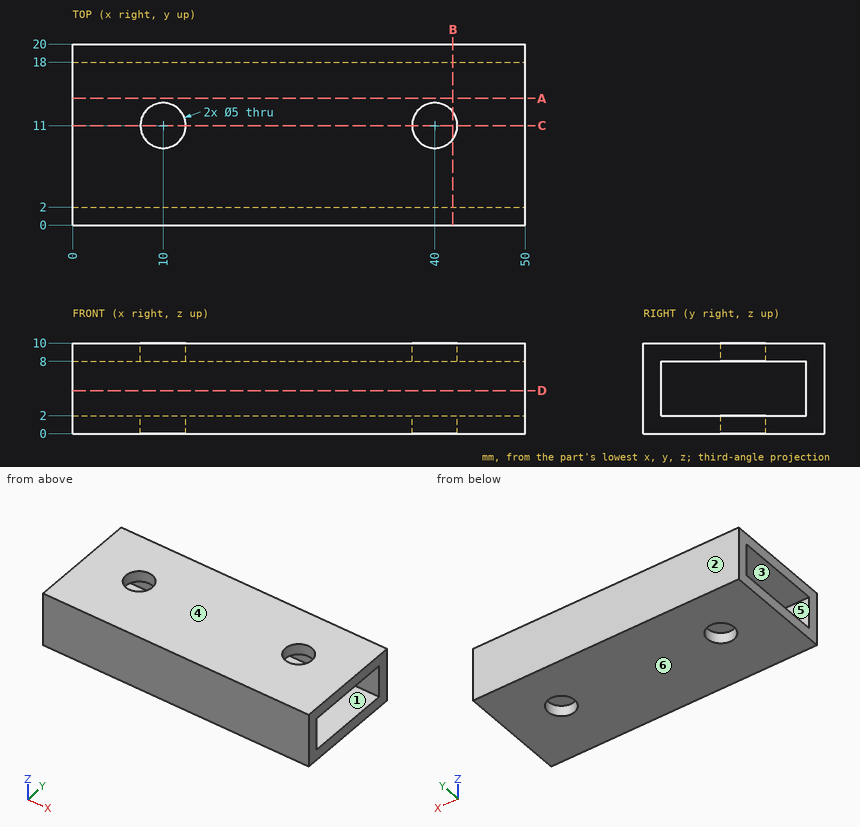
Geometry check sheet. Reference: drawing and pictorial views, mm from the part's lowest x, y, z. A direction names the side the tool comes from. Give positions to 0.01 mm unless a question says otherwise; leave off trailing zeros. Loops run counter-clockwise (first coordinate to the right, second up) from the corner with the lowest first, then second, coordinate; pieces in that order, holes last.
1. Section check B-B, the plane x = 42. Enter the section's corners in (y, z).
2. Thickness scan on line 1 (X direction, y = 11, z = 9.15); line 2 (Y direction, x = 17, z = 4.25); line 3 (Z direction, x = 46, y = 8). Record the ranges inside material, lowest first.
3. Mould release check, pull along Y, two halves, no side actions. Record for the marked faces 1, 2, 3 and 4: released by +Y, released by -Y, zero draft, split by the parting line, or undercut.
4. Section check D-D, the plane z = 4.75. Enter the section's corners in (x, y).
5. Go/stop test with a flat-tipped pin: pin 1 Ø10 at (x, y) = (12, 10) entering from -Z. Record where the tip stops, or that it passes through.
6. Section check C-C, the plane y = 11. Enter the section's corners in (x, z), then the cut area to 3 significant figures.
7. Set-up check for the marked faces 5 and 6: record each of +Z, -Z, +X, -X, +Y, -Y from which the full face is reachable in a straight line by a thin tool's end or side.
8. Section check A-A, the plane y = 14. Enter the section's corners in (x, z), then the cut area to 3 significant figures.
Geometry says:
1. outline: (0, 0) - (9.5, 0) - (9.5, 2) - (2, 2) - (2, 8) - (9.5, 8) - (9.5, 10) - (0, 10) - close; (12.5, 0) - (20, 0) - (20, 10) - (12.5, 10) - (12.5, 8) - (18, 8) - (18, 2) - (12.5, 2) - close
2. line 1: x = 0 to 7.5, 12.5 to 37.5, 42.5 to 50
2. line 2: y = 0 to 2, 18 to 20
2. line 3: z = 0 to 2, 8 to 10
3. face 1: undercut
3. face 2: released by +Y
3. face 3: undercut
3. face 4: zero draft
4. outline: (0, 0) - (50, 0) - (50, 2) - (0, 2) - close; (0, 18) - (50, 18) - (50, 20) - (0, 20) - close
5. pin 1: stops at z = 0
6. outline: (0, 0) - (7.5, 0) - (7.5, 2) - (0, 2) - close; (0, 8) - (7.5, 8) - (7.5, 10) - (0, 10) - close; (12.5, 0) - (37.5, 0) - (37.5, 2) - (12.5, 2) - close; (12.5, 8) - (37.5, 8) - (37.5, 10) - (12.5, 10) - close; (42.5, 0) - (50, 0) - (50, 2) - (42.5, 2) - close; (42.5, 8) - (50, 8) - (50, 10) - (42.5, 10) - close
6. area: 160 mm2
7. face 5: +X, -X
7. face 6: -Z, +X, -X, +Y, -Y
8. outline: (0, 0) - (50, 0) - (50, 2) - (0, 2) - close; (0, 8) - (50, 8) - (50, 10) - (0, 10) - close
8. area: 200 mm2
